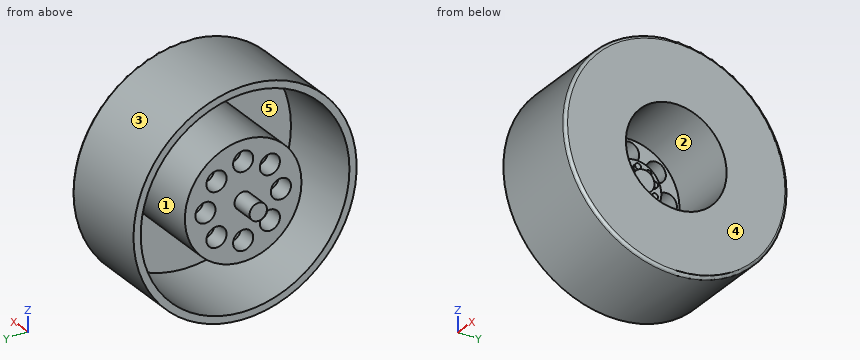
```python
from build123d import *

# Parameters (mm, degrees)
F0_R      = 19.685
F1_DEPTH  = 16.51
F2_R      = 8.89
F3_DEPTH  = 12.7
F4_R      = 4.445
F5_DEPTH  = 1.905
F6_R      = 1.905
F7_DEPTH  = 2.032
F8_R      = 1.778
F9_DEPTH  = 5.08
F10_R     = 0.508
F11_DEPTH = 0.508
F12_R     = 1.524
F13_DEPTH = 3.556
F14_R     = 10.287
F14_R_2   = 1.778
F14_R_3   = 1.524
F15_DEPTH = 0.508
F16_R     = 18.415
F16_R_2   = 10.287
F17_DEPTH = 15.748
F18_R     = 0.508


with BuildPart() as f1:
    # F0 (on Right) → F1 (new body)
    with BuildSketch(Plane.YZ):
        Circle(F0_R)
    extrude(amount=F1_DEPTH)

    # F2 (on face) → F3 (cut)
    with BuildSketch(Plane.YZ.offset(16.51)):
        Circle(F2_R)
    extrude(amount=-F3_DEPTH, mode=Mode.SUBTRACT)

    # F4 (on face) → F5 (join)
    with BuildSketch(Plane.YZ.offset(3.81)):
        Circle(F4_R)
    extrude(amount=F5_DEPTH)

    # F6 (on face) → F7 (join)
    with BuildSketch(Plane.YZ.offset(5.715)):
        Circle(F6_R)
    extrude(amount=F7_DEPTH)

    # F8 (on face) → F9 (cut)
    with BuildSketch(Plane.YZ.offset(3.81)):
        with Locations((0, 6.6575121996)):
            Circle(F8_R)
        with Locations((-4.7075720221, 4.7075720221)):
            Circle(F8_R)
        with Locations((-6.6575121996, 0)):
            Circle(F8_R)
        with Locations((-4.7075720221, -4.7075720221)):
            Circle(F8_R)
        with Locations((0, -6.6575121996)):
            Circle(F8_R)
        with Locations((4.7075720221, -4.7075720221)):
            Circle(F8_R)
        with Locations((6.6575121996, 0)):
            Circle(F8_R)
        with Locations((4.7075720221, 4.7075720221)):
            Circle(F8_R)
    extrude(amount=-F9_DEPTH, mode=Mode.SUBTRACT)

    # F10 (on face) → F11 (join)
    with BuildSketch(Plane.YZ.offset(5.715)):
        with Locations((0, 3.175)):
            Circle(F10_R)
        with Locations((-1.866218176, 2.5686289571)):
            Circle(F10_R)
        with Locations((-3.0196044392, 0.9811289571)):
            Circle(F10_R)
        with Locations((-3.0196044392, -0.9811289571)):
            Circle(F10_R)
        with Locations((-1.866218176, -2.5686289571)):
            Circle(F10_R)
        with Locations((0, -3.175)):
            Circle(F10_R)
        with Locations((1.866218176, -2.5686289571)):
            Circle(F10_R)
        with Locations((3.0196044392, -0.9811289571)):
            Circle(F10_R)
        with Locations((3.0196044392, 0.9811289571)):
            Circle(F10_R)
        with Locations((1.866218176, 2.5686289571)):
            Circle(F10_R)
    extrude(amount=F11_DEPTH)

    # F12 (on face) → F13 (join)
    with BuildSketch(Plane(origin=(0, 0, 0), x_dir=(0, -1, 0), z_dir=(-1, 0, 0))):
        Circle(F12_R)
    extrude(amount=F13_DEPTH)

    # F14 (on face) → F15 (cut)
    with BuildSketch(Plane(origin=(0, 0, 0), x_dir=(0, -1, 0), z_dir=(-1, 0, 0))):
        Circle(F14_R)
        with Locations((-4.7075720221, -4.7075720221)):
            Circle(F14_R_2, mode=Mode.SUBTRACT)
        with Locations((0, -6.6575121996)):
            Circle(F14_R_2, mode=Mode.SUBTRACT)
        with Locations((4.7075720221, -4.7075720221)):
            Circle(F14_R_2, mode=Mode.SUBTRACT)
        with Locations((-6.6575121996, 0)):
            Circle(F14_R_2, mode=Mode.SUBTRACT)
        with Locations((-4.7075720221, 4.7075720221)):
            Circle(F14_R_2, mode=Mode.SUBTRACT)
        Circle(F14_R_3, mode=Mode.SUBTRACT)
        with Locations((4.7075720221, 4.7075720221)):
            Circle(F14_R_2, mode=Mode.SUBTRACT)
        with Locations((6.6575121996, 0)):
            Circle(F14_R_2, mode=Mode.SUBTRACT)
        with Locations((0, 6.6575121996)):
            Circle(F14_R_2, mode=Mode.SUBTRACT)
    extrude(amount=-F15_DEPTH, mode=Mode.SUBTRACT)

    # F16 (on face) → F17 (cut)
    with BuildSketch(Plane(origin=(0, 0, 0), x_dir=(0, -1, 0), z_dir=(-1, 0, 0))):
        Circle(F16_R)
        Circle(F16_R_2, mode=Mode.SUBTRACT)
    extrude(amount=-F17_DEPTH, mode=Mode.SUBTRACT)

    # F18
    f18_edges = [f1.edges().sort_by_distance(p)[0] for p in [
        (16.51, -19.685, 0),
    ]]
    fillet(f18_edges, radius=F18_R)


solid = f1.part
```
Can you work these out from the model? Positions are in its coordinate system, mm. Face numbers are marked on the shaded views. A direction names the side the tool comes from. Give positions to 0.01 mm unless a question says otherwise; leave off trailing zeros. Answer in a Markdown table with one row per item.
1. Which directions (+Z, -Z, +X, -X, +Y, -Y) give clear straight access to the entire face, cutting with the end or side of a thin tool? Please do the marked faces 1 and 2.
Taken from the geometry:
| item | result |
|---|---|
| face 1 | -X |
| face 2 | +X |
2. Suppose I cut it at A-A on x = 3. Count the separate pieces of the cut face and the enclosed holes in it, plus the area to 3 significant figures.
Taken from the geometry:
| item | result |
|---|---|
| separate pieces | 2 |
| enclosed holes | 9 |
| area | 405 mm² |
3. If I drill on line 1 along Y through (x, z) = (1.75, 1); line 2 along Y through (x, z) = (10.5, -1.5); line 3 along X through (y, z) = (6.5, -9), over which ranges is the centre line in solid material (lowest first)?
Taken from the geometry:
| item | result |
|---|---|
| line 1 | y = -19.66 to -18.39, -10.24 to -8.13, -5.19 to 5.19, 8.13 to 10.24, 18.39 to 19.66 |
| line 2 | y = -19.63 to -18.35, -10.18 to -8.76, 8.76 to 10.18, 18.35 to 19.63 |
| line 3 | x = 15.75 to 16.51 |
4. Thinking about a two-plate mould opening in Z: for the marked faces 3, 4 and 5, which applies, released by +Z, released by -Z, zero draft, split by the parting line, or undercut?
Taken from the geometry:
| item | result |
|---|---|
| face 3 | split by the parting line |
| face 4 | zero draft |
| face 5 | undercut |
5. For pin 1 Ø1.9 at (y, z) = (-0.5, 0.5) entering from +X; pin 2 Ø3 at (x, y) = (10.5, 4.5) entering from +Z; pin 3 Ø8 at (x, y) = (13, 14) entering from +Z; pin 4 Ø2 at (y, z) = (4.71, -4.71) entering from +X, each with a flat end and sliding along its axis, tell me the tip position at first contact or that it passes through.
Taken from the geometry:
| item | result |
|---|---|
| pin 1 | stops at x = 7.75 |
| pin 2 | stops at z = 19.46 |
| pin 3 | stops at z = 16.96 |
| pin 4 | passes through |
